Drawing for the job (mm, zero at the part's lowest x, y, z). A direction names the side the tool comes from. Round coordinates to 2 decimals unless told otherwise and drop trailing zeros. Write each loop counter-clockwise with the first axis right and the second up, starting at its lowest first coordinate (ties: lowest second). Pieces come first, ordered by that corner, then holes. Notation, with made-up numbers: M 0.5,11 L 37.5,11 A18 cw 37.5,31 Z; hole C 66.5,86 d3. An arc over 180 degrees is marked long. Use a Markdown table: item, result. Add a question column.
1) Wall check: probe 1 along Y at (x, z) = (30, 10.5); probe 2 along Z at (x, y) = (9.5, 21); probe 3 along X at (y, z) = (20.5, 1.25) (1 decimal). Give the ranges that are in metal, low to high.
2) Slice it at C-C on x = 18. Write the cut outline in (y, z) (1 decimal), plus the area to 3 significant figures.
3) Slice it at B-B on y = 27.5. Write the cut outline in (x, z).
4) Drop flat-ended pins along their axis: P1, Ø12, axis at y = 9.5, z = 13.5, coming from the +X side (1 decimal); P2, Ø6, axis at y = 28, z = 4, coming from the +X side; P3, Ø10, axis at y = 30.5, z = 8.5, coming from the +X side. Give the stop position or say it passes through.
5) Which spindle directions (+Z, -Z, +X, -X, +Y, -Y) get a long thin tool onto all of the face, cutting with end or side? Do the marked faces 1 and 2. Say none if no direction does.
6) Slice it at A-A on z = 14.25. Write the cut outline in (x, y), plus the area to 3 significant figures.
7) Slice it at D-D on y = 4.5. Write the cut outline in (x, z).
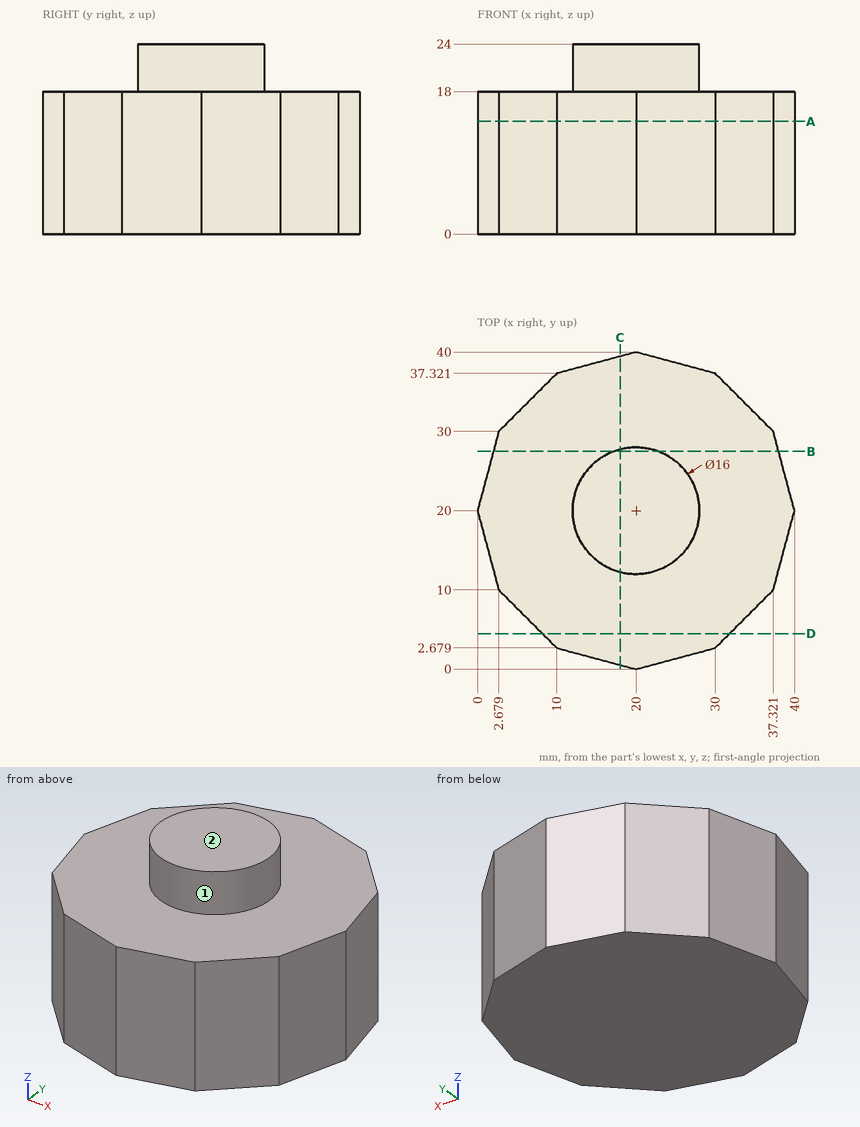
Entries:
| question | item | result |
|---|---|---|
| 1 | probe 1 | y = 2.68 to 37.32 |
| 1 | probe 2 | z = 0 to 18 |
| 1 | probe 3 | x = 0.1 to 39.9 |
| 2 | outline | M 0.5,0 L 39.5,0 L 39.5,18 L 27.7,18 L 27.7,24 L 12.3,24 L 12.3,18 L 0.5,18 Z |
| 2 | area | 794 mm^2 |
| 3 | outline | M 2.01,0 L 37.99,0 L 37.99,18 L 22.78,18 L 22.78,24 L 17.22,24 L 17.22,18 L 2.01,18 Z |
| 4 | P1 | stops at x = 38.8 |
| 4 | P2 | stops at x = 38.66 |
| 4 | P3 | stops at x = 38.53 |
| 5 | face 1 | +Z |
| 5 | face 2 | +Z, +X, -X, +Y, -Y |
| 6 | outline | M 0,20 L 2.68,10 L 10,2.68 L 20,0 L 30,2.68 L 37.32,10 L 40,20 L 37.32,30 L 30,37.32 L 20,40 L 10,37.32 L 2.68,30 Z |
| 6 | area | 1,200 mm^2 |
| 7 | outline | M 8.18,0 L 31.82,0 L 31.82,18 L 8.18,18 Z |
